from build123d import *

# Parameters (mm, degrees)
SKETCH3_R           = 12.5
BOSS_EXTRUDE2_DEPTH = 5
BOSS_EXTRUDE3_DEPTH = 9


with BuildPart() as part:
    # Sketch3 → Boss-Extrude2 (new, symmetric)
    # profile 1 of 4: a face of its own
    with BuildSketch(Plane.XY):
        with Locations((-36.682238028, -21.1785)):
            Circle(SKETCH3_R)
    # profile 2 of 4: a face of its own
    with BuildSketch(Plane.XY):
        with Locations((36.682238028, -21.1785)):
            Circle(SKETCH3_R)
    # profile 3 of 4: a face of its own
    with BuildSketch(Plane.XY):
        with Locations((0, 42.357)):
            Circle(SKETCH3_R)
    # profile 4 of 4: a face of its own
    with BuildSketch(Plane.XY):
        Polygon((0, 52.357), (-45.342492066, 26.1785), (-45.342492066, -26.1785), (0, -52.357), (45.342492066, -26.1785), (45.342492066, 26.1785), align=None)
        Polygon((0, 32.357), (-28.02198399, 16.1785), (-28.02198399, -16.1785), (0, -32.357), (28.02198399, -16.1785), (28.02198399, 16.1785), align=None, mode=Mode.SUBTRACT)
    extrude(amount=BOSS_EXTRUDE2_DEPTH, both=True)

    # Sketch4 → Boss-Extrude3 (add)
    with BuildSketch(Plane(origin=(0, 0, -5), x_dir=(-1, 0, 0), z_dir=(0, 0, -1))):
        Polygon((-41.332238028, -23.863178752), (-36.682238028, -26.547857503), (-32.032238028, -23.863178752), (-32.032238028, -18.493821248), (-36.682238028, -15.809142497), (-41.332238028, -18.493821248), align=None)
        Polygon((41.332238028, -23.863178752), (41.332238028, -18.493821248), (36.682238028, -15.809142497), (32.032238028, -18.493821248), (32.032238028, -23.863178752), (36.682238028, -26.547857503), align=None)
        Polygon((0, 47.726357503), (-4.65, 45.041678752), (-4.65, 39.672321248), (0, 36.987642497), (4.65, 39.672321248), (4.65, 45.041678752), align=None)
    extrude(amount=BOSS_EXTRUDE3_DEPTH)


solid = part.part
Source: CAD feature listing. Evaluate the final solid. Frame: model axes, mm. A direction names the side the tool comes from. Give positions to 0.01 mm unless a question says otherwise; leave off trailing zeros. Write each loop counter-clockwise with the first axis right and the second up, starting at its lowest first coordinate (ties: lowest second). Pieces come first, ordered by that corner, then holes. Notation, with made-up numbers: M -19,15 L 22,15 A20 cw 22,40 Z; hole C 32.25,-14 d2. An arc over 180 degrees is marked long. Answer as a JSON object with one key per item and string values.
Q1. Cut plane B-B, the plane z = 3.25. Return the cut outline in (x, y).
Geometry check:
{"outline": "M -45.34,-12.16 A12.5 ccw -33.21,-33.19 L 0,-52.36 L 33.21,-33.19 A12.5 ccw 45.34,-12.16 L 45.34,26.18 L 12.14,45.35 A12.5 ccw -12.14,45.35 L -45.34,26.18 Z; hole M -28.02,-12.16 A12.5 cw -24.55,-18.19 L 0,-32.36 L 24.55,-18.19 A12.5 cw 28.02,-12.16 L 28.02,16.18 L 3.48,30.35 A12.5 cw -3.48,30.35 L -28.02,16.18 Z"}
Q2. Cut plane C-C, the plane x = -6. Return the cut outline in (y, z), then the cut area to 3 significant figures.
Geometry check:
{"outline": "M -48.89,-5 L -28.89,-5 L -28.89,5 L -48.89,5 Z; M 28.89,-5 L 53.32,-5 L 53.32,5 L 28.89,5 Z", "area": "444 mm^2"}
Q3. Cut plane D-D, the plane x = -35. Return the cut outline in (y, z).
Geometry check:
{"outline": "M -33.56,-5 L -25.58,-5 L -25.58,-14 L -16.78,-14 L -16.78,-5 L 32.15,-5 L 32.15,5 L -33.56,5 Z"}
Q4. Contact query for flat-ended pins moving along their axis: P1, Ø2.5, axis at y = -20.5, z = -8, coming from the -X side; P2, Ø2, axis at x = 29, y = 18.5, coming from the -Z side; P3, Ø1.6, axis at y = -22, z = -8.5, coming from the +X side; P4, Ø5, axis at y = -20, z = -3, coming from the -X side. Output: stop coordinate, or through.
Geometry check:
{"P1": "stops at x = -41.33", "P2": "stops at z = -5", "P3": "stops at x = 41.33", "P4": "stops at x = -49.18"}
Q5. Ray query, line 1 along X through (y, z) = (5, 1); line 2 along Y through (x, z) = (-23.5, 2.5); line 3 along Z through (x, y) = (-15, -34.5). Return the intervals inside material, ascending.
Geometry check:
{"line 1": "x = -45.34 to -28.02, 28.02 to 45.34", "line 2": "y = -38.79 to -18.79, 18.79 to 38.79", "line 3": "z = -5 to 5"}
Q6. Cut plane A-A, the plane y = 1.5. Return the cut outline in (x, z).
Geometry check:
{"outline": "M -45.34,-5 L -28.02,-5 L -28.02,5 L -45.34,5 Z; M 28.02,-5 L 45.34,-5 L 45.34,5 L 28.02,5 Z"}
Q7. Mould query, pull axis X, two halves, no side actions, for faces 1 (the face through (28.022, 2, 0)), 2 (the face through (37, -21, -14)), 3 (the face through (-28.507, 35.898, 0.07)). Classes: +X half, -X half, draft (parallel to the pull), parting line (faces both ways), or undercut.
Geometry check:
{"face 1": "undercut", "face 2": "draft", "face 3": "-X half"}
Q8. Access query for faces 4 (the face through (34, -25, -9)), 5 (the face through (-4.65, 42, -9)), 6 (the face through (39.04, -25.187, -9.437)), 7 (the face through (12.1, -25.37, 0.07)). Directions: +Z, -Z, +X, -X, +Y, -Y. A direction counts if a zero-diameter tool reaches every point of the face in a straight line with its end or side. Return the directions, or none.
Geometry check:
{"face 4": "-Z, -Y", "face 5": "-Z, -X, +Y, -Y", "face 6": "-Z, +X, -Y", "face 7": "+Z, -Z"}
